Source: three-view drawing plus pictorial views. Frame: mm from the lowest corner of the part. A direction names the side the tool comes from. Coordinates: 2 decimals unless noted, no trailing zeros. Loops run counter-clockwise (first coordinate to the right, second up) from the corner with the lowest first, then second, coordinate; pieces in that order, holes last. Notation, with made-up numbers: (28.25, 5.25) - (38.25, 5.25) arc R5 cw to (38.25, 12.25) - close; hole circle Ø3 at (12, 84). An arc over 180 degrees is marked (long way). Return JSON: item names as keys, results as strings.
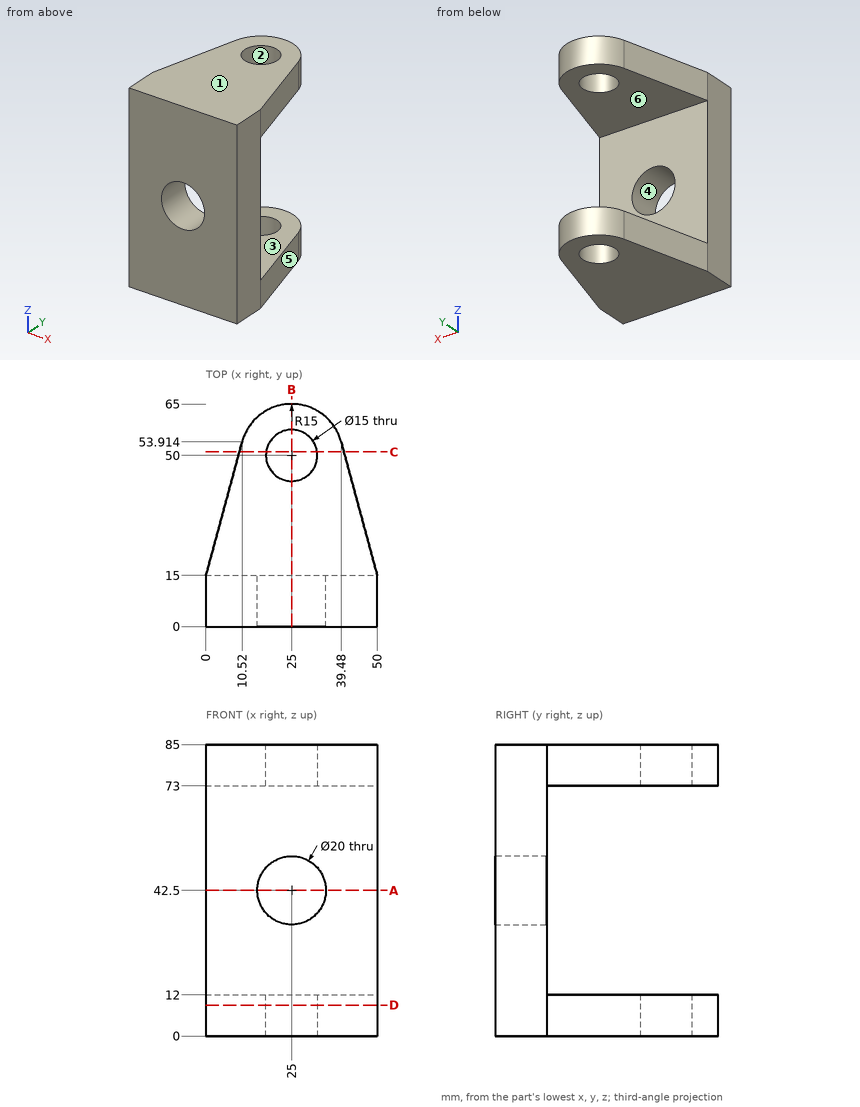
Item 1: Mould query, pull axis Z, two halves, no side actions, for the marked faces 1, 2, 3 and 4. Classes: +Z half, -Z half, draft (parallel to the pull), parting line (faces both ways), or undercut.
Worked out:
{"face 1": "+Z half", "face 2": "draft", "face 3": "undercut", "face 4": "undercut"}
Item 2: Section query B-B, the plane x = 25. Return loops of the section in (y, z), and give its area (4 significant figures).
Worked out:
{"outline": "(0, 0) - (42.5, 0) - (42.5, 12) - (15, 12) - (15, 32.5) - (0, 32.5) - close; (0, 52.5) - (15, 52.5) - (15, 73) - (42.5, 73) - (42.5, 85) - (0, 85) - close; (57.5, 0) - (65, 0) - (65, 12) - (57.5, 12) - close; (57.5, 73) - (65, 73) - (65, 85) - (57.5, 85) - close", "area": "1,815 mm^2"}
Item 3: Reachability of the marked faces 5 and 6 from +Z, -Z, +X, -X, +Y, -Y: full face, straight path, thin tool, end or side. Return the list, or none.
Worked out:
{"face 5": "+Z, -Z, +X, +Y", "face 6": "+X, -X, +Y"}
Item 4: First-contact query: pin 1 Ø6 at (x, y) = (21.5, 12) entering from -Z; pin 2 Ø8 at (x, z) = (6, 62.5) entering from +Y; pin 3 Ø1 at (y, z) = (18, 74) entering from -X (1 decimal). Flat tips, straight axial feed; report the tip coordinate or a pass-through.
Worked out:
{"pin 1": "z = 0", "pin 2": "y = 15", "pin 3": "x = 0.7"}
Item 5: Ray query, probe 1 along Z at (x, y) = (12, 52); probe 2 along X at (y, z) = (9, 42.5); probe 3 along Y at (x, z) = (43.5, 39.5). Return the intervals inside material, ascending. Write a range as from..to.
Worked out:
{"probe 1": "0..12, 73..85", "probe 2": "0..15, 35..50", "probe 3": "0..15"}
Item 6: Section query D-D, the plane z = 9. Return loops of the section in (x, y) (1 decimal).
Worked out:
{"outline": "(0, 0) - (50, 0) - (50, 15) - (39.5, 53.9) arc R15 ccw to (10.5, 53.9) - (0, 15) - close; hole circle Ø15 at (25, 50)"}
Item 7: Section query A-A, the plane z = 42.5. Return loops of the section in (x, y), and give its area (3 significant figures).
Worked out:
{"outline": "(0, 0) - (15, 0) - (15, 15) - (0, 15) - close; (35, 0) - (50, 0) - (50, 15) - (35, 15) - close", "area": "450 mm^2"}
Item 8: Section query C-C, the plane y = 51. Return loops of the section in (x, z).
Worked out:
{"outline": "(9.73, 0) - (17.57, 0) - (17.57, 12) - (9.73, 12) - close; (9.73, 73) - (17.57, 73) - (17.57, 85) - (9.73, 85) - close; (32.43, 0) - (40.27, 0) - (40.27, 12) - (32.43, 12) - close; (32.43, 73) - (40.27, 73) - (40.27, 85) - (32.43, 85) - close"}
